Source: CAD feature listing. Evaluate the final solid. Frame: model axes, mm. A direction names the side the tool comes from. Round coordinates to 2 decimals unless told otherwise and drop trailing zeros. Loops run counter-clockwise (first coordinate to the right, second up) from the corner with the lowest first, then second, coordinate; pieces in that order, holes last. Notation, with made-up numbers: M 11.5,3.25 L 69.5,3.25 A30 ccw 69.5,42.25 Z; hole C 27,23.25 d9. An arc over 180 degrees is marked long. Write each question's results on one line, items separated by ' | '. Start each with the question number.
1. Contact query for flat-ended pins moving along their axis: pin 1 Ø2 at (x, z) = (-55.5, 10) entering from +Y; pin 2 Ø2.5 at (x, z) = (-54.99, 4.52) entering from -Y. Output: stop coordinate, or through.
2. Set-up query: faces 1 (the cylindrical face through (-54.64, 48.1, 2.93)), 2 (the cylindrical face through (-52.81, 46.65, 10.59)), 3 (the flat face through (-55, 45, 8.273)). Return all of +Z, -Z, +X, -X, +Y, -Y with unobstructed straight access to the full face (end or side cutting, diameter ignored); none if empty.
3. Ray query, line 1 (X direction, y = 44.5, z = 5.5); line 2 (Z direction, x = -57.75, y = 42.75); line 3 (Z direction, x = -53, y = 45). Return the intervals inside material, ascending.
4. Draft query along X for faces 4 (the flat face through (-59.049, 45, 5)), 5 (the flat face through (-55, 47.924, 5)), 6 (the flat face through (-55, 46, 11.6)), 7 (the flat face through (-51.195, 45, 5)). Return one class per face: released by +X, released by -X, zero draft, split by the parting line, or undercut.
5. Section C-C on x = -54.75. Output: boundary loops of the cut face in (y, z), and give its area (3 significant figures).
6. Section D-D on z = 7.25. Output: boundary loops of the cut face in (x, y), and give its area (3 significant figures).
7. Section B-B on z = 5.5. Output: boundary loops of the cut face in (x, y).
8. Section A-A on y = 43.25. Output: boundary loops of the cut face in (x, z), and give its area (3 significant figures).
from build123d import *

# Parameters (mm, degrees)
F0_W     = 7.854256779
F0_H     = 6.4445212483
F1_DEPTH = 9.6
F2_R     = 2.4271283895
F3_DEPTH = 2
F4_W     = 5.3872168064
F4_H     = 5.2361704875
F5_DEPTH = 6
F6_R     = 2.0273342164
F6_R_2   = 1.6301233672
F7_DEPTH = 1


with BuildPart() as f1:
    # F0 (on Top) → F1 (new body)
    with BuildSketch(Plane.XY):
        with Locations((-55.12210913, 45.146599412)):
            Rectangle(F0_W, F0_H)
    extrude(amount=F1_DEPTH)

    # F2 (on face) → F3 (join)
    with BuildSketch(Plane.XY.offset(9.6)):
        with Locations((-55.12210913, 45.918174088)):
            Circle(F2_R)
    extrude(amount=F3_DEPTH)

    # F4 (on face) → F5 (cut)
    with BuildSketch(Plane.XZ.offset(-41.9243387878)):
        with Locations((-55.1610887051, 5.6545048719)):
            Rectangle(F4_W, F4_H)
    extrude(amount=-F5_DEPTH, mode=Mode.SUBTRACT)

    # F6 (on face) → F7 (cut)
    with BuildSketch(Plane(origin=(0, 48.3688600361, 0), x_dir=(-1, 0, 0), z_dir=(0, 1, 0))):
        with Locations((54.9886859953, 4.5204013586)):
            Circle(F6_R)
        with Locations((54.9886859953, 4.5204013586)):
            Circle(F6_R_2, mode=Mode.SUBTRACT)
    extrude(amount=-F7_DEPTH, mode=Mode.SUBTRACT)


solid = f1.part
Taken from the geometry:
1) pin 1: y = 48.37 | pin 2: y = 47.92
2) face 1: +Y | face 2: +Z | face 3: -Y
3) line 1: -59.05 to -57.85, -52.47 to -51.19 | line 2: 0 to 3.04, 8.27 to 9.6 | line 3: 0 to 3.04, 8.27 to 11.6
4) face 4: released by -X | face 5: undercut | face 6: zero draft | face 7: released by +X
5) outline: M 41.92,0 L 48.37,0 L 48.37,2.51 L 47.37,2.51 L 47.37,2.91 L 48.37,2.91 L 48.37,6.13 L 47.92,6.13 L 47.92,3.04 L 41.92,3.04 Z; M 41.92,8.27 L 47.92,8.27 L 47.92,6.53 L 48.37,6.53 L 48.37,9.6 L 48.32,9.6 L 48.32,11.6 L 43.52,11.6 L 43.52,9.6 L 41.92,9.6 Z | area: 39.5 mm^2
6) outline: M -59.05,41.92 L -57.85,41.92 L -57.85,47.92 L -52.47,47.92 L -52.47,41.92 L -51.19,41.92 L -51.19,48.37 L -59.05,48.37 Z | area: 18.3 mm^2
7) outline: M -59.05,41.92 L -57.85,41.92 L -57.85,47.92 L -56.76,47.92 L -56.76,48.37 L -59.05,48.37 Z; M -56.29,47.92 L -53.69,47.92 L -53.69,48.37 L -56.29,48.37 Z; M -53.21,47.92 L -52.47,47.92 L -52.47,41.92 L -51.19,41.92 L -51.19,48.37 L -53.21,48.37 Z
8) outline: M -59.05,0 L -51.19,0 L -51.19,9.6 L -59.05,9.6 Z; hole M -57.85,3.04 L -52.47,3.04 L -52.47,8.27 L -57.85,8.27 Z | area: 47.2 mm^2
